```python
from build123d import *

# Parameters (mm, degrees)
SKETCH1_R           = 47.5
BOSS_EXTRUDE1_DEPTH = 20
FILLET1_R           = 45
FILLET2_R           = 5


with BuildPart() as part:
    # Sketch1 → Boss-Extrude1 (new body)
    with BuildSketch(Plane.XY):
        Polygon((-99.803538153, -268.977427834), (188.085436338, -268.977427834), (188.085436338, -341.607655446), (244.140949093, -299.966804473), (244.140949093, -268.977427834), (244.140949093, 31.022572166), (44.140949093, 393.998813233), (-155.859050907, 31.022572166), (-155.859050907, -268.977427834), (-155.859050907, -299.966804473), (-99.803538153, -341.607655446), align=None)
        with Locations((44.140949093, -62.521501175)):
            Circle(SKETCH1_R, mode=Mode.SUBTRACT)
        Polygon((-125.859050907, -170.021501175), (-82.349617269, -170.021501175), (-125.859050907, -228.592437053), align=None, mode=Mode.SUBTRACT)
        Polygon((6.643511339, -250.596190725), (-53.211415944, -170.021501175), (141.493314129, -170.021501175), (81.638386846, -250.596190725), align=None, mode=Mode.SUBTRACT)
        Polygon((184.483743739, -238.977427834), (127.641085844, -238.977427834), (156.062414792, -200.717590916), align=None, mode=Mode.SUBTRACT)
        Polygon((-125.859050907, -140.021501175), (-82.349617269, -140.021501175), (-82.349617269, -90.186397517), (-82.349617269, -47.519598178), (-82.349617269, 14.978498825), (-125.859050907, 14.978498825), (-125.859050907, -47.519598178), (-125.859050907, -90.186397517), align=None, mode=Mode.SUBTRACT)
        Polygon((29.800552112, 255.428707564), (-21.612263577, 178.30948403), (29.800552112, 178.30948403), align=None, mode=Mode.SUBTRACT)
        Polygon((188.085436338, 61.022572166), (128.063188969, 151.05594322), (73.913154487, 61.022572166), align=None, mode=Mode.SUBTRACT)
        Polygon((-99.803538153, 61.022572166), (14.368743698, 61.022572166), (-39.781290784, 151.05594322), align=None, mode=Mode.SUBTRACT)
        Polygon((214.140949093, -228.592437053), (170.631515454, -170.021501175), (214.140949093, -170.021501175), align=None, mode=Mode.SUBTRACT)
        Polygon((214.140949093, -140.021501175), (214.140949093, -90.186397517), (214.140949093, -47.519598178), (214.140949093, 14.978498825), (170.631515454, 14.978498825), (170.631515454, -47.519598178), (170.631515454, -90.186397517), (170.631515454, -140.021501175), align=None, mode=Mode.SUBTRACT)
        Polygon((-96.201845554, -238.977427834), (-39.359187659, -238.977427834), (-67.780516606, -200.717590916), align=None, mode=Mode.SUBTRACT)
        with BuildLine():
            Line((-61.485967642, 14.978498825), (-61.485967642, -38.366786979))
            Line((-61.485967642, -38.366786979), (-29.498712654, -38.366786979))
            ThreePointArc((-29.498712654, -38.366786979), (-12.737505242, -9.880343963), (14.368743698, 9.03173625))
            Line((14.368743698, 9.03173625), (14.368743698, 14.978498825))
            Line((14.368743698, 14.978498825), (-61.485967642, 14.978498825))
        make_face(mode=Mode.SUBTRACT)
        with BuildLine():
            Line((-61.485967642, -140.021501175), (-61.485967642, -85.255349829))
            Line((-61.485967642, -85.255349829), (-29.949685439, -85.255349829))
            ThreePointArc((-29.949685439, -85.255349829), (-13.241152292, -114.6131938), (14.368743698, -134.074738599))
            Line((14.368743698, -134.074738599), (14.368743698, -140.021501175))
            Line((14.368743698, -140.021501175), (-61.485967642, -140.021501175))
        make_face(mode=Mode.SUBTRACT)
        with BuildLine():
            Line((73.913154487, -134.074738599), (73.913154487, -140.021501175))
            Line((73.913154487, -140.021501175), (149.767865827, -140.021501175))
            Line((149.767865827, -140.021501175), (149.767865827, -85.255349829))
            Line((149.767865827, -85.255349829), (118.231583625, -85.255349829))
            ThreePointArc((118.231583625, -85.255349829), (101.523050478, -114.6131938), (73.913154487, -134.074738599))
        make_face(mode=Mode.SUBTRACT)
        with BuildLine():
            Line((73.913154487, 9.03173625), (73.913154487, 14.978498825))
            Line((73.913154487, 14.978498825), (149.767865827, 14.978498825))
            Line((149.767865827, 14.978498825), (149.767865827, -38.366786979))
            Line((149.767865827, -38.366786979), (117.780610839, -38.366786979))
            ThreePointArc((117.780610839, -38.366786979), (101.019403427, -9.880343963), (73.913154487, 9.03173625))
        make_face(mode=Mode.SUBTRACT)
        Polygon((108.124840655, 162.105125634), (58.481346073, 162.105125634), (58.481346073, 79.564621072), align=None, mode=Mode.SUBTRACT)
        Polygon((109.894161762, 178.30948403), (58.481346073, 255.428707564), (58.481346073, 178.30948403), align=None, mode=Mode.SUBTRACT)
        Polygon((-19.84294247, 162.105125634), (29.800552112, 79.564621072), (29.800552112, 162.105125634), align=None, mode=Mode.SUBTRACT)
    extrude(amount=BOSS_EXTRUDE1_DEPTH)

    # Fillet1
    fillet1_edges = [part.edges().sort_by_distance(p)[0] for p in [
        (244.140949093, -299.966804473, 10),
        (-155.859050907, -299.966804473, 10),
        (-155.859050907, 31.022572166, 10),
        (44.140949093, 393.998813233, 10),
        (244.140949093, 31.022572166, 10),
    ]]
    fillet(fillet1_edges, radius=FILLET1_R)

    # Fillet2
    fillet2_edges = [part.edges().sort_by_distance(p)[0] for p in [
        (188.085436338, -341.607655446, 10),
        (-99.803538153, -341.607655446, 10),
    ]]
    fillet(fillet2_edges, radius=FILLET2_R)


solid = part.part
```
Geometry: final body of the model. Coordinates: model frame, mm. A direction names the side the tool comes from. Give positions to 0.01 mm unless a question says otherwise; leave off trailing zeros. Loops run counter-clockwise (first coordinate to the right, second up) from the corner with the lowest first, then second, coordinate; pieces in that order, holes last. Notation, with made-up numbers: (-24.5, -8) -> (3.5, -8) arc R28 cw to (3.5, 22) -> close; hole circle Ø1 at (-16.75, 72). An arc over 180 degrees is marked (long way). Return JSON: item names as keys, results as strings.
Item 1: Pin query (flat end, axial travel): P1, Ø10, axis at x = -40.5, z = 5.5, coming from the -Y side; P2, Ø6, axis at y = 140.5, z = 10.5, coming from the +X side; P3, Ø5, axis at y = 175, z = 10.5, coming from the +X side. Return the tip coordinate at first contact, or that it passes through.
Filled in:
{"P1": "y = -268.98", "P2": "x = 185.47", "P3": "x = 166.19"}
Item 2: Section A-A, the plane x = 163. Output: boundary loops of the cut face in (y, z).
Filled in:
{"outline": "(-268.98, 0) -> (-238.98, 0) -> (-238.98, 20) -> (-268.98, 20) -> close; (-210.06, 0) -> (61.02, 0) -> (61.02, 20) -> (-210.06, 20) -> close; (98.65, 0) -> (178.28, 0) -> (178.28, 20) -> (98.65, 20) -> close"}
Item 3: Line query: line 1 (X direction, y = 117, z = 13); line 2 (Y direction, x = 136, z = 8); line 3 (Y direction, x = -87, z = 7.5). Output: solid intervals per line, ascending.
Filled in:
{"line 1": "-108.49 to -62.49, -19.3 to 7.29, 29.8 to 58.48, 81 to 107.58, 150.77 to 196.77", "line 2": "-268.98 to -238.98, -227.72 to -177.42, -170.02 to -140.02, -85.26 to -38.37, 14.98 to 61.02, 139.15 to 227.29", "line 3": "-268.98 to -238.98, -226.59 to -176.28, -170.02 to -140.02, 14.98 to 61.02, 80.23 to 155.99"}
Item 4: Mould query, pull axis Y, two halves, no side actions, for faces 4 (the cylindrical face through (-150.929, -297.816, 10.14)), 5 (the flat face through (156, -238.977, 10)), 6 (the flat face through (41, 9, 20)). Classes: released by +Y, released by -Y, zero draft, split by the parting line, or undercut.
Filled in:
{"face 4": "released by -Y", "face 5": "undercut", "face 6": "zero draft"}
Item 5: Section C-C, the plane y = 206.5. Output: boundary loops of the cut face in (x, z).
Filled in:
{"outline": "(-59.17, 0) -> (-2.82, 0) -> (-2.82, 20) -> (-59.17, 20) -> close; (29.8, 0) -> (58.48, 0) -> (58.48, 20) -> (29.8, 20) -> close; (91.1, 0) -> (147.45, 0) -> (147.45, 20) -> (91.1, 20) -> close"}
Item 6: Section D-D, the plane y = -50. Output: boundary loops of the cut face in (x, z).
Filled in:
{"outline": "(-155.86, 0) -> (-125.86, 0) -> (-125.86, 20) -> (-155.86, 20) -> close; (-82.35, 0) -> (-1.68, 0) -> (-1.68, 20) -> (-82.35, 20) -> close; (89.96, 0) -> (170.63, 0) -> (170.63, 20) -> (89.96, 20) -> close; (214.14, 0) -> (244.14, 0) -> (244.14, 20) -> (214.14, 20) -> close"}
Item 7: Access query for faces 1 (the flat face through (244.141, -131, 10)), 2 (the flat face through (-61.486, -113, 10)), 3 (the flat face through (-99.804, -301, 10)). Directions: +Z, -Z, +X, -X, +Y, -Y. A direction counts if a zero-diameter tool reaches every point of the face in a straight line with its end or side. Return the directions, or none.
Filled in:
{"face 1": "+Z, -Z, +X, +Y, -Y", "face 2": "+Z, -Z", "face 3": "+Z, -Z, -Y"}
Item 8: Section B-B, the plane y = -295. Output: boundary loops of the cut face in (x, z), plus the area to 3 significant figures.
Filled in:
{"outline": "(-152.25, 0) -> (-99.8, 0) -> (-99.8, 20) -> (-152.25, 20) -> close; (188.09, 0) -> (240.53, 0) -> (240.53, 20) -> (188.09, 20) -> close", "area": "2,100 mm^2"}
